CAD build for the part. Positions are in the model's coordinates, mm. Coordinates: 2 decimals unless noted, no trailing zeros. Write each loop counter-clockwise with the first axis right and the second up, starting at its lowest first coordinate (ties: lowest second). Pieces come first, ordered by that corner, then holes. Notation, with made-up numbers: (-38.5, -28.75) - (-29.5, -28.75) arc R17 cw to (-29.5, 2.25) - close; hole circle Ø7 at (27.25, 27.5). An arc over 180 degrees is marked (long way). Answer in a Markdown table with one row per item. Add a question column.
Q1. Pin check, flat tips, straight feed: pin 1 (3 mm diameter, centred on x = -14, y = 1.5, fed in from -Z); pin 2 (8 mm diameter, centred on x = 174.5, z = 4, fed in from +Y). Stop position of each tip, or through.
Q2. Band-saw the part on A-A (y = 3.25). List the corners of the cut face in (x, z), and give its area (3 significant figures).
Q3. Band-saw the part on C-C (x = -42). List the corners of the cut face in (y, z).
Q4. Band-saw the part on B-B (z = 230.5). List the corners of the cut face in (x, y).
Q5. Two-plate mould, pull along X, no slides. Class faces 1 (the flat face through (4, 0, 7)), 2 (the flat face through (4, 0.5, 7)): +X half, -X half, draft (parallel to the pull), parting line (faces both ways), or undercut.
Q6. Drill centre lines: line 1 along X through (y, z) = (1, 393); line 2 along Y through (x, z) = (-206.5, -275.5). Where is each one in solid material? Low to high. Write a range as from..to.
Autodesk Inventor part; units mm, degrees
ref_plane "YZ Plane" through (0, 0, 0) normal (1, 0, 0) x (0, 1, 0)
ref_plane "XZ Plane" through (0, 0, 0) normal (0, 1, 0) x (-1, 0, 0)
ref_plane "XY Plane" through (0, 0, 0) normal (0, 0, 1) x (1, 0, 0)
sketch "Sketch6" plane through (0, 0, 0) normal (0, 1, 0) x (-1, 0, 0)
  line L0 (255.9, -490) -> (-255.9, -490)
  line L1 (-255.9, -490) -> (-255.9, 490)
  line L2 (-255.9, 490) -> (255.9, 490)
  line L3 (255.9, 490) -> (255.9, -490)
  line L4 (255.9, -490) -> (-255.9, 490) construction
  line L5 (-255.9, -490) -> (255.9, 490) construction
  point P0 (0, 0)
  dimension "d52" = 511.8
  dimension "d53" = 980
extrude "Plate2" add sketch "Sketch6" along normal blind 0.5
sketch "Sketch11" plane through (-255.4, 0, 490) normal (-1, 0, 0) x (0, -1, 0)
  line L0 (0, -980) -> (0, 0)
  line L1 (0, 0) -> (-10, 0)
  line L2 (-10, 0) -> (-10, -980)
  line L3 (-10, -980) -> (0, -980)
edge flange "Flange2" height 10 angle 90 thickness 0.5 bend radius 0.5 thickness toward (-1, 0, 0) relief tear relief width 0.5 relief depth 0.25 edges at (-255.9, 0.5, 0) wall of the first edge with corners at (-255.4, 0, -490) (-255.4, 0, 490) (-255.4, 10, 490) (-255.4, 10, -490)
bend "Bend3"
corner "Corner3"
sketch "Sketch12" plane through (-255.9, 9.5, 490) normal (0, 1, 0) x (-1, 0, 0)
  line L0 (0, -980) -> (0, 0)
  line L1 (0, 0) -> (-10, 0)
  line L2 (-10, 0) -> (-10, -980)
  line L3 (-10, -980) -> (0, -980)
edge flange "Flange3" height 10 angle 90 thickness 0.5 bend radius 0.5 thickness toward (0, 1, 0) relief tear relief width 0.5 relief depth 0.25 edges at (-255.4, 10, 0) wall of the first edge with corners at (-255.9, 9.5, -490) (-255.9, 9.5, 490) (-245.9, 9.5, 490) (-245.9, 9.5, -490)
bend "Bend4"
corner "Corner4"
sketch "Sketch13" plane through (255.4, 0, -490) normal (1, 0, 0) x (0, 1, 0)
  line L0 (0, 980) -> (0, 0)
  line L1 (0, 0) -> (10, 0)
  line L2 (10, 0) -> (10, 980)
  line L3 (10, 980) -> (0, 980)
edge flange "Flange4" height 10 angle 90 thickness 0.5 bend radius 0.5 thickness toward (1, 0, 0) relief tear relief width 0.5 relief depth 0.25 edges at (255.9, 0.5, 0) wall of the first edge with corners at (255.4, 0, 490) (255.4, 0, -490) (255.4, 10, -490) (255.4, 10, 490)
bend "Bend5"
corner "Corner5"
sketch "Sketch14" plane through (255.9, 9.5, -490) normal (0, 1, 0) x (-1, 0, 0)
  line L0 (0, 980) -> (0, 0)
  line L1 (0, 0) -> (10, 0)
  line L2 (10, 0) -> (10, 980)
  line L3 (10, 980) -> (0, 980)
edge flange "Flange5" height 10 angle 90 thickness 0.5 bend radius 0.5 thickness toward (0, 1, 0) relief tear relief width 0.5 relief depth 0.25 edges at (255.4, 10, 0) wall of the first edge with corners at (255.9, 9.5, 490) (255.9, 9.5, -490) (245.9, 9.5, -490) (245.9, 9.5, 490)
bend "Bend6"
corner "Corner6"
equation "\"d52\" = ЖАБРЫ_базовая_ширина - 4 * ЖАБРЫ_шаг_листов"
equation "\"d53\" = ЖАБРЫ_базовая_длина_кор_лист"
equation "\"d54\" = Thickness"
equation "\"d84\" = BendReliefWidth"
equation "\"d85\" = BendReliefDepth"
equation "\"d86\" = MinimumRemnant"
equation "\"d87\" = TransitionRadius"
equation "\"d90\" = BendRadius"
equation "\"d91\" = CornerReliefSize"
equation "\"d92\" = GapSize"
equation "\"d93\" = JacobiRadiusSize"
equation "\"d94\" = BendReliefWidth"
equation "\"d95\" = BendReliefDepth"
equation "\"d96\" = MinimumRemnant"
equation "\"d97\" = TransitionRadius"
equation "\"d100\" = BendRadius"
equation "\"d101\" = CornerReliefSize"
equation "\"d102\" = GapSize"
equation "\"d103\" = JacobiRadiusSize"
equation "\"d104\" = BendReliefWidth"
equation "\"d105\" = BendReliefDepth"
equation "\"d106\" = MinimumRemnant"
equation "\"d107\" = TransitionRadius"
equation "\"d110\" = BendRadius"
equation "\"d111\" = CornerReliefSize"
equation "\"d112\" = GapSize"
equation "\"d113\" = JacobiRadiusSize"
equation "\"d114\" = BendReliefWidth"
equation "\"d115\" = BendReliefDepth"
equation "\"d116\" = MinimumRemnant"
equation "\"d117\" = TransitionRadius"
equation "\"d120\" = BendRadius"
equation "\"d121\" = CornerReliefSize"
equation "\"d122\" = GapSize"
equation "\"d123\" = JacobiRadiusSize"
equation "\"BendRadius\" = Thickness"
equation "\"BendReliefWidth\" = Thickness"
equation "\"BendReliefDepth\" = 0.5 * Thickness"
equation "\"CornerReliefSize\" = 4 * Thickness"
equation "\"MinimumRemnant\" = 2 * Thickness"
equation "\"TransitionRadius\" = BendRadius"
equation "\"JacobiRadiusSize\" = BendRadius"
equation "\"GapSize\" = Thickness"
properties part number "MSC 809 sheet gills" material "Stainless Steel"
Checked values:
| question | item | result |
|---|---|---|
| 1 | pin 1 | stops at z = -490 |
| 1 | pin 2 | stops at y = 0.5 |
| 2 | outline | (-255.9, -490) - (-255.4, -490) - (-255.4, 490) - (-255.9, 490) - close; (255.4, -490) - (255.9, -490) - (255.9, 490) - (255.4, 490) - close |
| 2 | area | 980 mm² |
| 3 | outline | (0, -490) - (0.5, -490) - (0.5, 490) - (0, 490) - close |
| 4 | outline | (-255.9, 1) arc R1 ccw to (-254.9, 0) - (254.9, 0) arc R1 ccw to (255.9, 1) - (255.9, 9) arc R1 ccw to (254.9, 10) - (245.9, 10) - (245.9, 9.5) - (254.9, 9.5) arc R0.5 cw to (255.4, 9) - (255.4, 1) arc R0.5 cw to (254.9, 0.5) - (-254.9, 0.5) arc R0.5 cw to (-255.4, 1) - (-255.4, 9) arc R0.5 cw to (-254.9, 9.5) - (-245.9, 9.5) - (-245.9, 10) - (-254.9, 10) arc R1 ccw to (-255.9, 9) - close |
| 5 | face 1 | draft |
| 5 | face 2 | undercut |
| 6 | line 1 | x = -255.9..-255.4, 255.4..255.9 |
| 6 | line 2 | y = 0..0.5 |
